Autodesk Inventor part; units mm, degrees
ref_plane "YZ Plane" through (0, 0, 0) normal (1, 0, 0) x (0, 1, 0)
ref_plane "XZ Plane" through (0, 0, 0) normal (0, 1, 0) x (-1, 0, 0)
ref_plane "XY Plane" through (0, 0, 0) normal (0, 0, 1) x (1, 0, 0)
sketch "Sketch1" plane through (0, 0, 0) normal (0, 1, 0) x (-1, 0, 0)
  line L0 (0, 0) -> (162.56, 0)
  line L1 (162.56, 0) -> (162.56, -210.82)
  line L2 (81.28, -292.1) -> (81.28, -292.1)
  line L3 (0, -210.82) -> (0, 0)
  arc A0 (81.28, -292.1) -> (162.56, -210.82) centre (81.28, -210.82) ccw
  arc A1 (0, -210.82) -> (81.28, -292.1) centre (81.28, -210.82) ccw
  point P0 (162.56, -292.1)
  point P1 (0, -292.1)
  dimension "d0" = 292.1
  dimension "d1" = 162.56
  dimension "d2" = 81.28
extrude "Extrusion1" add sketch "Sketch1" along normal blind 73.66
sketch "Sketch2" plane through (0, 73.66, 0) normal (0, 1, 0) x (1, 0, 0)
  line L0 (-162.56, 0) -> (0, 0)
  line L1 (0, 0) -> (0, 210.82)
  line L2 (-162.56, 0) -> (0, 0)
  line L3 (0, 0) -> (0, 96.52)
  line L4 (0, 96.52) -> (-162.56, 96.52)
  line L5 (-162.56, 96.52) -> (-162.56, 0)
  dimension "d23" = 114.3
extrude "Extrusion2" add sketch "Sketch2" along normal blind 388.62
sketch "Sketch3" plane through (-162.56, 0, 0) normal (0, 0, 1) x (1, 0, 0)
  line L0 (162.56, 0) -> (0, 0)
  line L1 (162.56, 0) -> (162.56, 462.28)
  line L2 (0, 0) -> (162.56, 0)
  line L3 (162.56, 0) -> (162.56, 431.8)
  line L4 (132.08, 462.28) -> (30.48, 462.28)
  line L5 (0, 431.8) -> (0, 0)
  arc A0 (30.48, 462.28) -> (0, 431.8) centre (30.48, 431.8) ccw
  arc A1 (162.56, 431.8) -> (132.08, 462.28) centre (132.08, 431.8) ccw
  dimension "d8" = 30.48
extrude "Extrusion3" cut sketch "Sketch3" against normal blind 508 keep common part
sketch "Sketch4" plane through (0, 73.66, -96.52) normal (0, 0, -1) x (-1, 0, 0)
  line L0 (132.08, 388.62) -> (30.48, 388.62)
  circle A0 centre (81.28, 313.69) radius 59.69
  line L1 (0, -73.66) -> (162.56, -73.66)
  dimension "d12" = 119.38
  dimension "d22" = 387.35
extrude "Extrusion4" add sketch "Sketch4" along normal blind 20.32
sketch "Sketch5" plane through (-81.28, 387.35, -116.84) normal (0, 0, -1) x (-1, 0, 0)
  circle A0 centre (0, 0) radius 30.48
  point P0 (-81.28, -387.35)
  dimension "d15" = 60.96
extrude "Extrusion5" add sketch "Sketch5" along normal blind 38.1
sketch "Sketch6" plane through (0, 0, 0) normal (0, -1, 0) x (1, 0, 0)
  arc A0 (-162.56, -210.82) -> (0, -210.82) centre (-81.28, -210.82) ccw
  circle A1 centre (-81.28, -210.82) radius 31.75
  point P0 (0, 0)
  dimension "d18" = 63.5
extrude "Extrusion6" cut sketch "Sketch6" against normal blind 25.4
properties part number "Waist Link"
Here's how the part is built. I have some questions about the finished solid (model axes, mm). A direction names the side the tool comes from. Give positions to 0.01 mm unless a question says otherwise; leave off trailing zeros. Loops run counter-clockwise (first coordinate to the right, second up) from the corner with the lowest first, then second, coordinate; pieces in that order, holes last. Notation, with made-up numbers: M -27.5,65 L 24.5,65 A10 ccw 24.5,79 Z; hole C -12,-4 d11. An arc over 180 degrees is marked long. Put each result on its own line as item: value. Start each with the question number.
(1) I want a section at D-D on z = -253. Please give me the cut outline in (x, y), then the cut area to 3 significant figures.
(2) Will this pin go through, and if not, where does the flat tip stop? pin 1 Ø2 at (x, z) = (-118, -223) entering from +Y.
(3) I want a section at B-B on x = -81.28. Please give me the cut outline in (y, z), then the cut area to 3 significant figures.
(4) I want a section at A-A on z = -108. Please give me the cut outline in (x, y), then the cut area to 3 significant figures.
(5) I need wall thicknesses on line 1 along X through (y, z) = (18, -210); line 2 along Z through (x, y) = (-81.28, 5); line 3 along Y through (x, z) = (-17, -97). Which ranges of each line are inside material? Lowest first, please. Write a range as [from, to].
(6) I want a section at C-C on y = 387.35. Please give me the cut outline in (x, z).
(7) If we mould it in two halves opening along Y, with no side actions, what happens to faces 1 (the flat face through (-67, 415, -116.84)), 2 (the flat face through (-80, 228, 0)), 3 (the cylindrical face through (-153.39, 453.59, -47.58))? For each: +Y half, -Y half, draft (parallel to the pull), parting line (faces both ways), or undercut.
(8) For faces 4 (the flat face through (0, 165, -60)), 5 (the cylindrical face through (-50.83, 386.01, -135.62)), 6 (the flat face through (-80, 73.66, -193)), 7 (the flat face through (-81, 388, -154.94)), 8 (the cylindrical face through (-66.63, 12.52, -238.99)), which set-ups out of +Z, -Z, +X, -X, +Y, -Y let a thin tool reach every point of the face, with its end or its side?
Answer block:
1. outline: M -150.76,0 L -11.8,0 L -11.8,73.66 L -150.76,73.66 Z
1. area: 10,200 mm^2
2. pin 1: y = 73.66
3. outline: M 0,-292.1 L 73.66,-292.1 L 73.66,-96.52 L 327.66,-96.52 L 327.66,-116.84 L 356.87,-116.84 L 356.87,-154.94 L 417.83,-154.94 L 417.83,-116.84 L 447.04,-116.84 L 447.04,-96.52 L 462.28,-96.52 L 462.28,0 L 0,0 L 0,-179.07 L 25.4,-179.07 L 25.4,-242.57 L 0,-242.57 Z
3. area: 62,200 mm^2
4. outline: M -162.56,0 L 0,0 L 0,73.66 L -162.56,73.66 Z; C -81.28,387.35 d119.38
4. area: 23,200 mm^2
5. line 1: [-162.56, -113.02], [-49.54, 0]
5. line 2: [-292.1, -242.57], [-179.07, 0]
5. line 3: [0, 73.66]
6. outline: M -162.56,-96.52 L -140.97,-96.52 L -140.97,-116.84 L -111.76,-116.84 L -111.76,-154.94 L -50.8,-154.94 L -50.8,-116.84 L -21.59,-116.84 L -21.59,-96.52 L 0,-96.52 L 0,0 L -162.56,0 Z
7. face 1: undercut
7. face 2: draft
7. face 3: +Y half
8. face 4: +Z, -Z, +X, +Y, -Y
8. face 5: -Z
8. face 6: -Z, +X, -X
8. face 7: -Z, +X, -X, +Y
8. face 8: -Y
